CAD build for the part. Positions are in the model's coordinates, mm. Face numbers are marked on the shaded views. Coordinates: 2 decimals unless noted, no trailing zeros. Loops run counter-clockwise (first coordinate to the right, second up) from the corner with the lowest first, then second, coordinate; pieces in that order, holes last. Notation, with made-up numbers: (47, -33) -> (55, -33) arc R17 ccw to (55, -14) -> close; hole circle Ø4 at (68, -22.75). An arc over 180 degrees is marked (long way). Write item = value, one per line. Start each with the question number.
(1) Band-saw the part on C-C (y = 203). Write the cut outline in (x, z), and give its area (3 significant figures).
(2) Drill centre lines: line 1 (X direction, y = 387, z = -23); line 2 (Z direction, x = -2, y = -413.5); line 3 (Z direction, x = 3.5, y = -248). Where is each one in solid material? Low to high. Write a range as from..to.
(3) Flat gauge pins, fed straight in: P1, Ø1, axis at x = 30.5, y = 295.5, coming from the +Z side; P2, Ø13, axis at y = 406.4, z = 0, coming from the -X side; P3, Ø4, axis at x = 20, y = -297.5, coming from the +Z side; P4, Ø4, axis at x = 41, y = 375, coming from the -Z side. Where does each tip first touch, or does it go through?
(4) Band-saw the part on A-A (y = 406.4). Write the cut outline in (x, z) (3 decimals), and give its area (3 significant figures).
(5) Band-saw the part on B-B (z = 26.5). Write the cut outline in (x, y), and give its area (3 significant figures).
(6) Band-saw the part on D-D (y = -133). Write the cut outline in (x, z).
(7) Pull direction X, two halves, no side cores. Call the marked faces 1, 2 and 3: +X half, -X half, draft (parallel to the pull), parting line (faces both ways), or undercut.
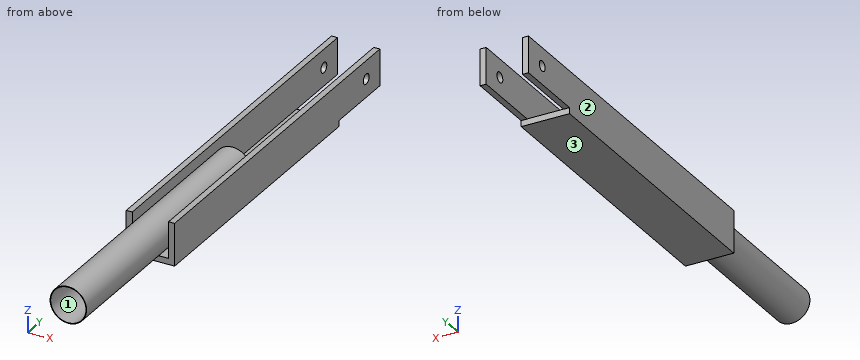
```python
from build123d import *

# Parameters (mm, degrees)
F0_R     = 38.1
F0_R_2   = 36.83
F1_DEPTH = 609.6
F2_W     = 12.7
F2_H     = 76.2
F3_DEPTH = 304.8
F4_DEPTH = 457.2
F5_W     = 101.092
F5_H     = 12.7
F6_DEPTH = 304.8
F7_DEPTH = 304.8
F8_R     = 10.795
F9_DEPTH = 50.8


with BuildPart() as f1:
    # F0 (on Front) → F1 (new body)
    with BuildSketch(Plane.XZ):
        Circle(F0_R)
        Circle(F0_R_2, mode=Mode.SUBTRACT)
    extrude(amount=F1_DEPTH)

    # F2 (on Front) → F3 (join)
    with BuildSketch(Plane.XZ):
        with Locations((44.196, 0)):
            Rectangle(F2_W, F2_H)
        with Locations((-44.196, 0)):
            Rectangle(F2_W, F2_H)
    extrude(amount=F3_DEPTH)

    # F2 (on Front) → F4 (join)
    with BuildSketch(Plane.XZ):
        with Locations((44.196, 0)):
            Rectangle(F2_W, F2_H)
        with Locations((-44.196, 0)):
            Rectangle(F2_W, F2_H)
    extrude(amount=-F4_DEPTH)

    # F5 (on Front) → F6 (join)
    with BuildSketch(Plane.XZ):
        with Locations((0, -44.196)):
            Rectangle(F5_W, F5_H)
    extrude(amount=F6_DEPTH)

    # F5 (on Front) → F7 (join)
    with BuildSketch(Plane.XZ):
        with Locations((0, -44.196)):
            Rectangle(F5_W, F5_H)
    extrude(amount=-F7_DEPTH)

    # F8 (on Right) → F9 (cut, symmetric)
    with BuildSketch(Plane.YZ):
        with Locations((406.4, 0)):
            Circle(F8_R)
    extrude(amount=F9_DEPTH, both=True, mode=Mode.SUBTRACT)


solid = f1.part
```
Findings below:
q1.outline = (-50.55, -50.55) -> (50.55, -50.55) -> (50.55, 38.1) -> (37.85, 38.1) -> (37.85, -37.85) -> (-37.85, -37.85) -> (-37.85, 38.1) -> (-50.55, 38.1) -> close
q1.area = 3,210 mm²
q2.line_1 = -50.55..-37.85, 37.85..50.55
q2.line_2 = -38.05..-36.78, 36.78..38.05
q2.line_3 = -50.55..-36.66, 36.66..37.94
q3.P1 = -37.85
q3.P2 = through
q3.P3 = 33.58
q3.P4 = -38.1
q4.outline = (-50.546, -38.1) -> (-37.846, -38.1) -> (-37.846, -10.795) -> (-50.546, -10.795) -> close; (-50.546, 10.795) -> (-37.846, 10.795) -> (-37.846, 38.1) -> (-50.546, 38.1) -> close; (37.846, -38.1) -> (50.546, -38.1) -> (50.546, -10.795) -> (37.846, -10.795) -> close; (37.846, 10.795) -> (50.546, 10.795) -> (50.546, 38.1) -> (37.846, 38.1) -> close
q4.area = 1,390 mm²
q5.outline = (-50.55, -304.8) -> (-37.85, -304.8) -> (-37.85, 457.2) -> (-50.55, 457.2) -> close; (-27.37, -609.6) -> (-25.58, -609.6) -> (-25.58, 0) -> (-27.37, 0) -> close; (25.58, -609.6) -> (27.37, -609.6) -> (27.37, 0) -> (25.58, 0) -> close; (37.85, -304.8) -> (50.55, -304.8) -> (50.55, 457.2) -> (37.85, 457.2) -> close
q5.area = 21,500 mm²
q6.outline = (-50.55, -50.55) -> (50.55, -50.55) -> (50.55, 38.1) -> (37.85, 38.1) -> (37.85, 4.39) arc R38.1 ccw to (-37.85, 4.39) -> (-37.85, 38.1) -> (-50.55, 38.1) -> close; hole (-37.85, -37.85) -> (-4.39, -37.85) arc R38.1 cw to (-37.85, -4.39) -> close; hole circle Ø73.66 at (0, 0); hole (4.39, -37.85) -> (37.85, -37.85) -> (37.85, -4.39) arc R38.1 cw to start
q7.face_1 = undercut
q7.face_2 = -X half
q7.face_3 = draft
